The listing builds one solid part. Answer for the finished solid, in the listing's coordinates (mm). Coordinates: 2 decimals unless noted, no trailing zeros. Write each loop counter-clockwise with the first axis right and the second up, starting at its lowest first coordinate (ties: lowest second). Pieces come first, ordered by that corner, then holes.
```python
from build123d import *

# Parameters (mm, degrees)
SKETCH1_R           = 16.5
BOSS_EXTRUDE1_DEPTH = 18
FILLET1_R           = 10
SKETCH2_R           = 6.5
BOSS_EXTRUDE2_DEPTH = 4
FILLET5_R           = 5


with BuildPart() as part:
    # Sketch1 → Boss-Extrude1 (new body)
    with BuildSketch(Plane(origin=(0, 0, 0), x_dir=(1, 0, 0), z_dir=(0, 1, 0))):
        with Locations(Location((0, 0, 0), (0, 0, 270))):
            Circle(SKETCH1_R)
    extrude(amount=BOSS_EXTRUDE1_DEPTH)

    # Fillet1
    fillet1_edges = [part.edges().sort_by_distance(p)[0] for p in [
        (0, 18, -16.5),
    ]]
    fillet(fillet1_edges, radius=FILLET1_R)

    # Sketch2 → Boss-Extrude2 (add)
    with BuildSketch(Plane(origin=(0, 18, 0), x_dir=(1, 0, 0), z_dir=(0, 1, 0))):
        with Locations(Location((0, 0, 0), (0, 0, 270))):
            Circle(SKETCH2_R)
    extrude(amount=BOSS_EXTRUDE2_DEPTH)

    # Fillet5
    # the kernel refuses this fillet: 5 mm, written as the material it takes off along each edge
    with BuildSketch(Plane(origin=(0, 22, 0), x_dir=(0, 0, 1), z_dir=(-1, 0, 0))) as fillet5_piece_1:
        with BuildLine():
            CenterArc((1.601020514, -5), FILLET5_R, 11.536959033, 78.463040967)
            Line((1.601020514, 0), (1.601020514, 0.1))
            Line((1.601020514, 0.1), (6.5, 0.1))
            Line((6.5, 0.1), (6.6, 0))
            ThreePointArc((6.6, 0), (6.6, -2), (6.59797959, -3.98))
            Line((6.59797959, -3.98), (6.5, -4))
        make_face()
    revolve(axis=Axis((0, 22, 0), (0, 1, 0)), mode=Mode.SUBTRACT)


solid = part.part
```
(1) Find the intervals of material crossed by probe 1 along Y at (x, z) = (-9, 4); probe 2 along Z at (x, y) = (4, 4); probe 3 along Z at (x, y) = (10, 8.25), in increasing order.
(2) Each of these flat-tipped pins is pushed along its axis until it touches: pin 1 (2 mm diameter, centred on y = 9, z = 12, fed in from +X); pin 2 (12 mm diameter, centred on x = 10.5, y = 13, fed in from -Z); pin 3 (5 mm diameter, centred on x = -5, z = -12.5, fed in from +Y); pin 4 (10 mm diameter, centred on x = -3, z = -9.5, fed in from -Y). Where does it stop, or does it pass through?
(3) Section A-A, the plane y = 3.5 is taken. Write down the section's boundary in (x, z), plus the area to 3 significant figures.
Solution:
1. probe 1: y = 0 to 17.42
1. probe 2: z = -16.01 to 16.01
1. probe 3: z = -13.12 to 13.12
2. pin 1: stops at x = 12.24
2. pin 2: stops at z = -15.41
2. pin 3: stops at y = 16.95
2. pin 4: stops at y = 0
3. outline: circle Ø33 at (0, 0)
3. area: 855 mm2
